Design review of the part built by this model. Coordinates are the model's own, in mm. Give positions to 0.01 mm unless a question says otherwise; leave off trailing zeros. Order: outer loops, then holes, each group sorted by start corner. A loop starts at its lowest first (then second) coordinate and runs counter-clockwise, first axis right, second up. Notation, with made-up numbers: M 64,5.25 L 96,5.25 A32 cw 96,37.25 Z; hole C 5,-40 d9. An arc over 180 degrees is marked long. Put each result on its own line as item: value. Start each with the question number.
from build123d import *

# Parameters (mm, degrees)
SKETCH_1_W             = 150
SKETCH_1_H             = 45.5
EXTRUDE_1_DEPTH        = 2
CUT_EXTRUDE_1_REACH    = 80.4
SKETCH_2_R             = 1.65
CHAMFER_1_SIZE         = 8
CUT_EXTRUDE_1137_REACH = 80.4
SKETCH_3_R             = 2.5
CUT_EXTRUDE_2_REACH    = 80.4
SKETCH_4_R             = 1.65


with BuildPart() as part:
    # Sketch 1 → Extrude 1 (new body)
    with BuildSketch(Plane(origin=(0, 0, 0), x_dir=(1, 0, 0), z_dir=(0, 1, 0))):
        Rectangle(SKETCH_1_W, SKETCH_1_H)
    extrude(amount=EXTRUDE_1_DEPTH)

    # Sketch 2 → Cut-Extrude 1 (cut, up to next)
    with BuildSketch(Plane(origin=(0, 2, 0), x_dir=(1, 0, 0), z_dir=(0, 1, 0)), mode=Mode.PRIVATE) as cut_extrude_1_sk1:
        with Locations(Location((-60, 15, 0), (0, 0, 270))):
            Circle(SKETCH_2_R)
    cut_extrude_1_tool1 = extrude(cut_extrude_1_sk1.sketch, amount=-CUT_EXTRUDE_1_REACH, mode=Mode.PRIVATE) & part.part
    # Sketch 2 → Cut-Extrude 1 (cut, up to next)
    with BuildSketch(Plane(origin=(0, 2, 0), x_dir=(1, 0, 0), z_dir=(0, 1, 0)), mode=Mode.PRIVATE) as cut_extrude_1_sk2:
        with Locations(Location((-66, 7, 0), (0, 0, 270))):
            Circle(SKETCH_2_R)
    cut_extrude_1_tool2 = extrude(cut_extrude_1_sk2.sketch, amount=-CUT_EXTRUDE_1_REACH, mode=Mode.PRIVATE) & part.part
    # Sketch 2 → Cut-Extrude 1 (cut, up to next)
    with BuildSketch(Plane(origin=(0, 2, 0), x_dir=(1, 0, 0), z_dir=(0, 1, 0)), mode=Mode.PRIVATE) as cut_extrude_1_sk3:
        with Locations(Location((-54, 7, 0), (0, 0, 270))):
            Circle(SKETCH_2_R)
    cut_extrude_1_tool3 = extrude(cut_extrude_1_sk3.sketch, amount=-CUT_EXTRUDE_1_REACH, mode=Mode.PRIVATE) & part.part
    # Sketch 2 → Cut-Extrude 1 (cut, up to next)
    with BuildSketch(Plane(origin=(0, 2, 0), x_dir=(1, 0, 0), z_dir=(0, 1, 0)), mode=Mode.PRIVATE) as cut_extrude_1_sk4:
        with Locations(Location((-71, -7, 0), (0, 0, 270))):
            Circle(SKETCH_2_R)
    cut_extrude_1_tool4 = extrude(cut_extrude_1_sk4.sketch, amount=-CUT_EXTRUDE_1_REACH, mode=Mode.PRIVATE) & part.part
    # Sketch 2 → Cut-Extrude 1 (cut, up to next)
    with BuildSketch(Plane(origin=(0, 2, 0), x_dir=(1, 0, 0), z_dir=(0, 1, 0)), mode=Mode.PRIVATE) as cut_extrude_1_sk5:
        with Locations(Location((-59, -7, 0), (0, 0, 270))):
            Circle(SKETCH_2_R)
    cut_extrude_1_tool5 = extrude(cut_extrude_1_sk5.sketch, amount=-CUT_EXTRUDE_1_REACH, mode=Mode.PRIVATE) & part.part
    # Sketch 2 → Cut-Extrude 1 (cut, up to next)
    with BuildSketch(Plane(origin=(0, 2, 0), x_dir=(1, 0, 0), z_dir=(0, 1, 0)), mode=Mode.PRIVATE) as cut_extrude_1_sk6:
        with Locations(Location((-65, -15, 0), (0, 0, 270))):
            Circle(SKETCH_2_R)
    cut_extrude_1_tool6 = extrude(cut_extrude_1_sk6.sketch, amount=-CUT_EXTRUDE_1_REACH, mode=Mode.PRIVATE) & part.part
    cut_extrude_1_1 = cut_extrude_1_tool1.solids().sort_by_distance((-60, 2, -15))[0]
    add(cut_extrude_1_1, mode=Mode.SUBTRACT)
    cut_extrude_1_2 = cut_extrude_1_tool2.solids().sort_by_distance((-66, 2, -7))[0]
    add(cut_extrude_1_2, mode=Mode.SUBTRACT)
    cut_extrude_1_3 = cut_extrude_1_tool3.solids().sort_by_distance((-54, 2, -7))[0]
    add(cut_extrude_1_3, mode=Mode.SUBTRACT)
    cut_extrude_1_4 = cut_extrude_1_tool4.solids().sort_by_distance((-71, 2, 7))[0]
    add(cut_extrude_1_4, mode=Mode.SUBTRACT)
    cut_extrude_1_5 = cut_extrude_1_tool5.solids().sort_by_distance((-59, 2, 7))[0]
    add(cut_extrude_1_5, mode=Mode.SUBTRACT)
    cut_extrude_1_6 = cut_extrude_1_tool6.solids().sort_by_distance((-65, 2, 15))[0]
    add(cut_extrude_1_6, mode=Mode.SUBTRACT)
    cut_extrude_1 = cut_extrude_1_1 + cut_extrude_1_2 + cut_extrude_1_3 + cut_extrude_1_4 + cut_extrude_1_5 + cut_extrude_1_6  # Cut-Extrude 1 as one shape, for the pattern or mirror that repeats it

    # Mirror 1: Cut-Extrude 1 across plane
    add(cut_extrude_1.mirror(Plane(origin=(0, 0, 0), x_dir=(0, 0, 1), z_dir=(1, 0, 0))), mode=Mode.SUBTRACT)

    # Chamfer 1
    chamfer_1_edges = [part.edges().sort_by_distance(p)[0] for p in [
        (75, 1, 22.75),
        (-75, 1, 22.75),
    ]]
    chamfer(chamfer_1_edges, length=CHAMFER_1_SIZE)

    # Sketch 3 → Cut-Extrude 1137 (cut, up to next)
    with BuildSketch(Plane(origin=(0, 2, 0), x_dir=(1, 0, 0), z_dir=(0, 1, 0)), mode=Mode.PRIVATE) as cut_extrude_1137_sk1:
        with Locations(Location((0, 0, 0), (0, 0, 270))):
            Circle(SKETCH_3_R)
    cut_extrude_1137_tool1 = extrude(cut_extrude_1137_sk1.sketch, amount=-CUT_EXTRUDE_1137_REACH, mode=Mode.PRIVATE) & part.part
    add(cut_extrude_1137_tool1.solids().sort_by_distance((0, 2, 0))[0], mode=Mode.SUBTRACT)

    # Sketch 4 → Cut-Extrude 2 (cut, up to next)
    with BuildSketch(Plane(origin=(0, 2, 0), x_dir=(1, 0, 0), z_dir=(0, 1, 0)), mode=Mode.PRIVATE) as cut_extrude_2_sk1:
        with Locations(Location((-40, 18, 0), (0, 0, 270))):
            Circle(SKETCH_4_R)
    cut_extrude_2_tool1 = extrude(cut_extrude_2_sk1.sketch, amount=-CUT_EXTRUDE_2_REACH, mode=Mode.PRIVATE) & part.part
    # Sketch 4 → Cut-Extrude 2 (cut, up to next)
    with BuildSketch(Plane(origin=(0, 2, 0), x_dir=(1, 0, 0), z_dir=(0, 1, 0)), mode=Mode.PRIVATE) as cut_extrude_2_sk2:
        with Locations(Location((-40, -18, 0), (0, 0, 270))):
            Circle(SKETCH_4_R)
    cut_extrude_2_tool2 = extrude(cut_extrude_2_sk2.sketch, amount=-CUT_EXTRUDE_2_REACH, mode=Mode.PRIVATE) & part.part
    # Sketch 4 → Cut-Extrude 2 (cut, up to next)
    with BuildSketch(Plane(origin=(0, 2, 0), x_dir=(1, 0, 0), z_dir=(0, 1, 0)), mode=Mode.PRIVATE) as cut_extrude_2_sk3:
        with Locations(Location((40, 18, 0), (0, 0, 270))):
            Circle(SKETCH_4_R)
    cut_extrude_2_tool3 = extrude(cut_extrude_2_sk3.sketch, amount=-CUT_EXTRUDE_2_REACH, mode=Mode.PRIVATE) & part.part
    # Sketch 4 → Cut-Extrude 2 (cut, up to next)
    with BuildSketch(Plane(origin=(0, 2, 0), x_dir=(1, 0, 0), z_dir=(0, 1, 0)), mode=Mode.PRIVATE) as cut_extrude_2_sk4:
        with Locations(Location((40, -18, 0), (0, 0, 270))):
            Circle(SKETCH_4_R)
    cut_extrude_2_tool4 = extrude(cut_extrude_2_sk4.sketch, amount=-CUT_EXTRUDE_2_REACH, mode=Mode.PRIVATE) & part.part
    add(cut_extrude_2_tool1.solids().sort_by_distance((-40, 2, -18))[0], mode=Mode.SUBTRACT)
    add(cut_extrude_2_tool2.solids().sort_by_distance((-40, 2, 18))[0], mode=Mode.SUBTRACT)
    add(cut_extrude_2_tool3.solids().sort_by_distance((40, 2, -18))[0], mode=Mode.SUBTRACT)
    add(cut_extrude_2_tool4.solids().sort_by_distance((40, 2, 18))[0], mode=Mode.SUBTRACT)


solid = part.part
1. Consider section A-A on z = 18. Give the boundary of the cut face in (x, y), then the cut area to 3 significant figures.
2. The part is to be moulded in two halves that separate along X. For faces 1 (the cylindrical face through (-67.6, 1, -7.4)), 2 (the flat face through (-1, 0, -5)), 3 (the flat face through (-70.94, 0.99, 18.81)), say which applies: +X half, -X half, draft (parallel to the pull), parting line (faces both ways), or undercut.
3. Insertion check: pin 1 (2.5 mm diameter, centred on x = -59, z = 7, fed in from +Y). The pin has a flat end and moves straight along its axis. Give the tip position at first contact, or say it passes through.
4. Consider section C-C on z = -7. Give the boundary of the cut face in (x, y).
5. To check wall thickness, follow probe 1 along X at (y, z) = (0.8, -15); probe 2 along X at (y, z) = (1, 7); probe 3 along X at (y, z) = (1.45, -18). State the ranges of each line that lie inside material, in increasing order.
6. Consider section B-B on x = -54. Give the boundary of the cut face in (y, z), then the cut area to 3 significant figures.
7. Consider section D-D on y = 1.45. Give the number of separate pieces and of enclosed holes in the cut face, then the cut area to 3 significant figures.
Returned:
1. outline: M -71.75,0 L -41.65,0 L -41.65,2 L -71.75,2 Z; M -38.35,0 L 38.35,0 L 38.35,2 L -38.35,2 Z; M 41.65,0 L 71.75,0 L 71.75,2 L 41.65,2 Z
1. area: 274 mm2
2. face 1: undercut
2. face 2: draft
2. face 3: -X half
3. pin 1: passes through
4. outline: M -75,0 L -67.65,0 L -67.65,2 L -75,2 Z; M -64.35,0 L -55.65,0 L -55.65,2 L -64.35,2 Z; M -52.35,0 L 52.35,0 L 52.35,2 L -52.35,2 Z; M 55.65,0 L 64.35,0 L 64.35,2 L 55.65,2 Z; M 67.65,0 L 75,0 L 75,2 L 67.65,2 Z
5. probe 1: x = -75 to -61.65, -58.35 to 58.35, 61.65 to 75
5. probe 2: x = -75 to -72.65, -69.35 to -60.65, -57.35 to 57.35, 60.65 to 69.35, 72.65 to 75
5. probe 3: x = -75 to -41.65, -38.35 to 38.35, 41.65 to 75
6. outline: M 0,-22.75 L 2,-22.75 L 2,-8.65 L 0,-8.65 Z; M 0,-5.35 L 2,-5.35 L 2,22.75 L 0,22.75 Z
6. area: 84.4 mm2
7. separate pieces: 1
7. enclosed holes: 17
7. area: 6,600 mm2
